```python
from build123d import *

# Parameters (mm, degrees)
SKETCH1_W                   = 80
SKETCH1_H                   = 50
BOSS_EXTRUDE1_DEPTH         = 200
SKETCH4_W                   = 40
SKETCH4_H                   = 50
SKETCH4_R                   = 10
BOSS_EXTRUDE3_DEPTH         = 5
FILLET1_RADIUS              = 25
FILLET1_LENGTH              = 5
FILLET1_OF_MIRROR1_2_RADIUS = 25
FILLET1_OF_MIRROR1_2_LENGTH = 5


with BuildPart() as part:
    # Sketch1 → Boss-Extrude1 (new body)
    with BuildSketch(Plane.XY):
        Rectangle(SKETCH1_W, SKETCH1_H)
    extrude(amount=-BOSS_EXTRUDE1_DEPTH)

    # Sketch4 → Boss-Extrude3 (add)
    with BuildSketch(Plane(origin=(40, 0, 0), x_dir=(0, 0, -1), z_dir=(1, 0, 0))):
        with Locations((-20, 0)):
            Rectangle(SKETCH4_W, SKETCH4_H)
        with Locations(Location((-20, 0, 0), (0, 0, 90))):
            Circle(SKETCH4_R, mode=Mode.SUBTRACT)
    boss_extrude3 = extrude(amount=-BOSS_EXTRUDE3_DEPTH)

    # Fillet1: full round fillet: the end face becomes a half cylinder, R = half its width
    fillet1_face = Plane((37.5, 0, 40), x_dir=(-1, 0, 0), z_dir=(0, 0, 1))  # on the end face: x along it, z out of the body
    fillet1_slab = fillet1_face.offset(-FILLET1_RADIUS / 2) * Box(FILLET1_LENGTH, 2 * FILLET1_RADIUS, FILLET1_RADIUS, mode=Mode.PRIVATE)  # the body's end, R deep
    fillet1_round = Plane((37.5, 0, 15), x_dir=(0, 0, 1), z_dir=(-1, 0, 0)) * Cylinder(FILLET1_RADIUS, FILLET1_LENGTH, mode=Mode.PRIVATE)  # its axis R under the face
    add(fillet1_slab - fillet1_round, mode=Mode.SUBTRACT)

    # Mirror1: Boss-Extrude3 across plane
    add(boss_extrude3.mirror(Plane(origin=(0, 0, 0), x_dir=(0, 0, 1), z_dir=(1, 0, 0))))

    # Fillet1 of Mirror1 2: full round fillet: the end face becomes a half cylinder, R = half its width
    fillet1_of_mirror1_2_face = Plane((-37.5, 0, 40), x_dir=(1, 0, 0), z_dir=(0, 0, 1))  # on the end face: x along it, z out of the body
    fillet1_of_mirror1_2_slab = fillet1_of_mirror1_2_face.offset(-FILLET1_OF_MIRROR1_2_RADIUS / 2) * Box(FILLET1_OF_MIRROR1_2_LENGTH, 2 * FILLET1_OF_MIRROR1_2_RADIUS, FILLET1_OF_MIRROR1_2_RADIUS, mode=Mode.PRIVATE)  # the body's end, R deep
    fillet1_of_mirror1_2_round = Plane((-37.5, 0, 15), x_dir=(0, 0, 1), z_dir=(1, 0, 0)) * Cylinder(FILLET1_OF_MIRROR1_2_RADIUS, FILLET1_OF_MIRROR1_2_LENGTH, mode=Mode.PRIVATE)  # its axis R under the face
    add(fillet1_of_mirror1_2_slab - fillet1_of_mirror1_2_round, mode=Mode.SUBTRACT)


solid = part.part
```
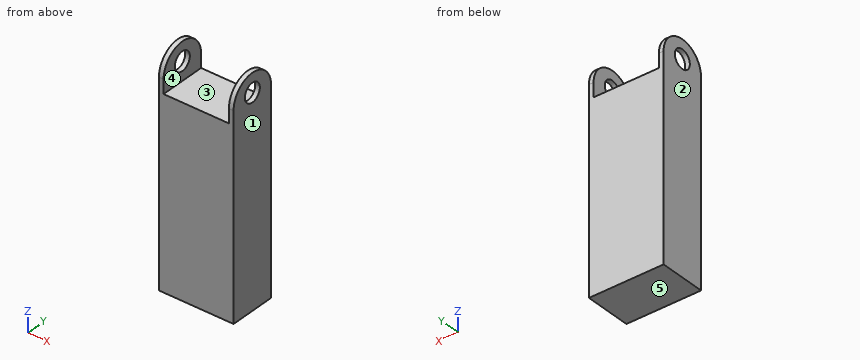
For this review, take the finished solid that the model builds, in its own axes (mm). Face numbers are marked on the shaded views. A direction names the side the tool comes from. Round coordinates to 2 decimals unless told otherwise and drop trailing zeros. Write each loop counter-clockwise with the first axis right and the second up, starting at its lowest first coordinate (ties: lowest second). Pieces come first, ordered by that corner, then holes. Notation, with made-up numbers: (51.25, -25) - (98.25, -25) arc R20 ccw to (98.25, 10) - close; hole circle Ø11 at (9.5, -33.75). An arc over 180 degrees is marked (long way). Put each result on its own line as item: value.
Q1. Mouldability with a two-part tool opening along X and no side actions: class the marked faces 1, 2 and 3 as released by +X, released by -X, zero draft, split by the parting line, or undercut.
Solved:
face 1: released by +X
face 2: released by -X
face 3: undercut
Q2. We need section C-C (y = -18.5). Give the boundary of the cut face in (x, z).
Solved:
outline: (-40, -200) - (40, -200) - (40, 31.82) - (35, 31.82) - (35, 0) - (-35, 0) - (-35, 31.82) - (-40, 31.82) - close
Q3. We need section A-A (y = 0). Give the boundary of the cut face in (x, z), and give its area (3 significant figures).
Solved:
outline: (-40, -200) - (40, -200) - (40, 10) - (35, 10) - (35, 0) - (-35, 0) - (-35, 10) - (-40, 10) - close; (-40, 30) - (-35, 30) - (-35, 40) - (-40, 40) - close; (35, 30) - (40, 30) - (40, 40) - (35, 40) - close
area: 16,200 mm2
Q4. Insertion check: pin 1 Ø1.5 at (x, y) = (28, -0.5) entering from +Z; pin 2 Ø16 at (y, z) = (0, 20) entering from +X. Each pin has a flat end and moves straight along its axis. Give the tip position at first contact, or say it passes through.
Solved:
pin 1: stops at z = 0
pin 2: passes through
Q5. Wall thickness on probe 1 along Z at (x, y) = (-37.3, 0); probe 2 along X at (y, z) = (-21.5, 16.5); probe 3 along Z at (x, y) = (25, -1.5): over which ranges is each line inside the solid? List them lowest first.
Solved:
probe 1: z = -200 to 10, 30 to 40
probe 2: x = -40 to -35, 35 to 40
probe 3: z = -200 to 0
Q6. We need section B-B (z = 20). Give the boundary of the cut face in (x, y), and give its area (3 significant figures).
Solved:
outline: (-40, -24.49) - (-35, -24.49) - (-35, -10) - (-40, -10) - close; (-40, 10) - (-35, 10) - (-35, 24.49) - (-40, 24.49) - close; (35, -24.49) - (40, -24.49) - (40, -10) - (35, -10) - close; (35, 10) - (40, 10) - (40, 24.49) - (35, 24.49) - close
area: 290 mm2
Q7. We need section D-D (x = -19.5). Give the boundary of the cut face in (y, z), and give its area (3 significant figures).
Solved:
outline: (-25, -200) - (25, -200) - (25, 0) - (-25, 0) - close
area: 10,000 mm2
Q8. Machinability: for the marked faces 4 and 5, which of the approach directions +Z, -Z, +X, -X, +Y, -Y give a long, thin tool a straight path to every point of the face, cutting with its end or side? Answer none if there is none.
Solved:
face 4: +Z, +Y, -Y
face 5: -Z, +X, -X, +Y, -Y
